Autodesk Inventor part; units mm, degrees
ref_plane "YZ Plane" through (0, 0, 0) normal (1, 0, 0) x (0, 1, 0)
ref_plane "XZ Plane" through (0, 0, 0) normal (0, 1, 0) x (-1, 0, 0)
ref_plane "XY Plane" through (0, 0, 0) normal (0, 0, 1) x (1, 0, 0)
sketch "Boceto1" plane through (0, 0, 0) normal (0, 1, 0) x (-1, 0, 0)
  circle A0 centre (0, 0) radius 8
  dimension "d0" = 16
extrude "Extrusión1" add sketch "Boceto1" along normal blind 21.6
sketch "Boceto2" plane through (0, 21.6, 0) normal (0, 1, 0) x (1, 0, 0)
  circle A0 centre (0, 0) radius 7.9
  dimension "d3" = 15.8
extrude "Extrusión2" add sketch "Boceto2" along normal blind 2.2
fillet "Empalme1" radius 1 1 edges at (-7.9, 23.8, 0)
sketch "Boceto3" plane through (0, 23.8, 0) normal (0, 1, 0) x (1, 0, 0)
  circle A0 centre (0, 0) radius 3
  circle A1 centre (0, 0) radius 1.75
  circle A2 centre (0, 0) radius 0.75
  dimension "d7" = 6
  dimension "d8" = 3.5
  dimension "d13" = 1.5
extrude "Extrusión3" add sketch "Boceto3" along normal blind 1 contours A0
extrude "Extrusión4" add sketch "Boceto3" along normal blind 2.1 contours A1 | A2
extrude "Extrusión5" add sketch "Boceto3" along normal blind 8.1 contours A2
sketch "Boceto4" plane through (0, 0, 0) normal (0, -1, 0) x (1, 0, 0)
  circle A0 centre (0, 0) radius 0.75
  circle A1 centre (0, 0) radius 6.5
  dimension "d16" = 13
extrude "Extrusión6" add sketch "Boceto4" along normal blind 1 contours A0 | A1
properties part number "Motor" material "Acero inoxidable"
Verification items for the finished model (mm, model axes). A direction names the side the tool comes from. Coordinates: 2 decimals unless noted, no trailing zeros. Write each loop counter-clockwise with the first axis right and the second up, starting at its lowest first coordinate (ties: lowest second). Pieces come first, ordered by that corner, then holes. Notation, with made-up numbers: M 66.25,40 L 95.25,40 A18 ccw 95.25,47 Z; hole C 1,36 d6. An arc over 180 degrees is marked long. One line per item, written item: value.
Item 1: Access from +Z, -Z, +X, -X, +Y, -Y to the whole of each face (thin tool, end or side, straight path). Record for faces 4 (the flat face through (0, 31.9, 0)), 5 (the cylindrical face through (-5.158, -0.493, 3.955)), 6 (the flat face through (0, 25.9, 1)).
Check sheet entries:
face 4: +Z, -Z, +X, -X, +Y
face 5: -Y
face 6: +Y
Item 2: Section check A-A, the plane x = 0. Record the boundary of the cut face in (y, z).
Check sheet entries:
outline: M -1,-6.5 L 0,-6.5 L 0,-8 L 21.6,-8 L 21.6,-7.9 L 22.8,-7.9 A1 ccw 23.8,-6.9 L 23.8,-3 L 24.8,-3 L 24.8,-1.75 L 25.9,-1.75 L 25.9,-0.75 L 31.9,-0.75 L 31.9,0.75 L 25.9,0.75 L 25.9,1.75 L 24.8,1.75 L 24.8,3 L 23.8,3 L 23.8,6.9 A1 ccw 22.8,7.9 L 21.6,7.9 L 21.6,8 L 0,8 L 0,6.5 L -1,6.5 Z
Item 3: Section check B-B, the plane z = 0. Record the boundary of the cut face in (x, y).
Check sheet entries:
outline: M -8,0 L -6.5,0 L -6.5,-1 L 6.5,-1 L 6.5,0 L 8,0 L 8,21.6 L 7.9,21.6 L 7.9,22.8 A1 ccw 6.9,23.8 L 3,23.8 L 3,24.8 L 1.75,24.8 L 1.75,25.9 L 0.75,25.9 L 0.75,31.9 L -0.75,31.9 L -0.75,25.9 L -1.75,25.9 L -1.75,24.8 L -3,24.8 L -3,23.8 L -6.9,23.8 A1 ccw -7.9,22.8 L -7.9,21.6 L -8,21.6 Z
Item 4: Scan lines: line 1 along Y through (x, z) = (1.25, -5.75); line 2 along Y through (x, z) = (6, -3.5); line 3 along X through (y, z) = (20, -0.25). Record each from-to range of solid material in increasing order.
Check sheet entries:
line 1: y = -1 to 23.8
line 2: y = 0 to 23.8
line 3: x = -8 to 8
Item 5: Section check C-C, the plane y = 15. Record the boundary of the cut face in (x, z).
Check sheet entries:
outline: C 0,0 d16
Item 6: Mould release check, pull along Y, two halves, no side actions. Record for faces 1 (the cylindrical face through (1.73, 10.65, 7.81)), 2 (the flat face through (3, 23.8, 1)), 3 (the flat face through (0, 0, 7)): pulls with the +Y half, pulls with the -Y half, needs draft (parallel to the pull), parting line crosses it, or undercut.
Check sheet entries:
face 1: needs draft
face 2: pulls with the +Y half
face 3: pulls with the -Y half
Item 7: Gauge pin test, flat ends, axial feed: pin 1 Ø3 at (y, z) = (27, 3) entering from -X; pin 2 Ø6 at (x, z) = (5, 6.5) entering from +Y; pin 3 Ø4 at (y, z) = (19.5, -5.5) entering from +X; pin 4 Ø6 at (x, y) = (3.5, 15.5) entering from -Z. Record the tip position at first contact, or that the pin passes through.
Check sheet entries:
pin 1: passes through
pin 2: stops at y = 23.8
pin 3: stops at x = 7.19
pin 4: stops at z = -7.98
